The listing builds one solid part. Answer for the finished solid, in the listing's coordinates (mm). A direction names the side the tool comes from. Round coordinates to 2 decimals unless told otherwise and drop trailing zeros. Write each loop counter-clockwise with the first axis right and the second up, starting at its lowest first coordinate (ties: lowest second). Pieces come first, ordered by that corner, then holes. Notation, with made-up numbers: (-29.75, 32.25) - (24.25, 32.25) arc R16 ccw to (24.25, 54.25) - close; hole circle Ø6 at (-34.5, 40.25). An arc over 180 degrees is marked (long way). Answer as CSV lines item,"result". Start each with the question number.
Item 1: Which of the six approach directions +Z, -Z, +X, -X, +Y, -Y give full straight-line access (tool end or side, diameter ignored) to faces 1 (the flat face through (69.167, -0.231, 39.005)), 2 (the flat face through (8, 19.05, 28)), 3 (the flat face through (-51.3, -0.23, 20.22))?
Item 2: A cutting plane is placed at C-C on z = 50.5. Determine the outline of the cut face in (x, y), and give its area (3 significant figures).
Item 3: For a pull along Y with two mould halves and no side action, classify faces 4 (the flat face through (8, -19.05, 29)), 5 (the flat face through (11.1, -0.27, 9.39)), 6 (the flat face through (8, 16.51, 29)), 7 (the flat face through (8, -16.51, 29)) as pulls with the +Y half, pulls with the -Y half, needs draft (parallel to the pull), parting line crosses it, or undercut.
Item 4: A cutting plane is placed at A-A on z = 17. Determine the outline of the cut face in (x, y).
Item 5: Straight lines are drawn through the part: line 1 along Y through (x, z) = (-25, 39); line 2 along X through (y, z) = (9.5, 35); line 3 along X through (y, z) = (-4.5, 33). For each, find the intervals that lie inside material, in ascending order. Write a range as [from, to].
Item 6: A cutting plane is placed at B-B on y = 2. Determine the outline of the cut face in (x, z) (3 decimals), and give its area (3 significant figures).
Item 7: A cutting plane is placed at D-D on z = 31. Determine the outline of the cut face in (x, y).
Item 8: Flat-ended cylindrical pins translate along their axes: pin 1 (1.5 mm diameter, centred on x = 32, y = -13, fed in from -Z); pin 2 (3 mm diameter, centred on x = -29.5, y = -0.5, fed in from -Z); pin 3 (6 mm diameter, centred on x = -29, y = 5, fed in from -Z). Find the tip coordinate at first contact, or state that the pin passes through.
```python
from build123d import *

# Parameters (mm, degrees)
F1_DEPTH = 19.05
F2_W     = 121.92
F2_H     = 2.54
F3_DEPTH = 35.56


with BuildPart() as f1:
    # F0 (on Front) → F1 (new body, symmetric)
    with BuildSketch(Plane.XZ):
        Polygon((-56.515, 37.6689364729), (-50.8, 0), (74.7631215764, 19.05), (69.0481215764, 56.7189364729), (66.5368591448, 56.3379364729), (71.8708591448, 21.1802624315), (-48.6697375685, 2.8922624315), (-54.0037375685, 38.0499364729), align=None)
    extrude(amount=F1_DEPTH, both=True)

    # F2 (on face) → F3 (join)
    with BuildSketch(Plane(origin=(-1.524, 0, 10.0450497261), x_dir=(0.9886859967, 0, 0.15), z_dir=(-0.15, 0, 0.9886859967))):
        with Locations((13.2747513695, 17.78)):
            Rectangle(F2_W, F2_H)
        with Locations((13.2747513695, -17.78)):
            Rectangle(F2_W, F2_H)
    extrude(amount=F3_DEPTH)


solid = f1.part
```
Geometry says:
1,face 1,"none"
1,face 2,"+Z, -Z, +X, -X, +Y"
1,face 3,"+Z"
2,outline,"(28.06, -19.05) - (69.99, -19.05) - (69.99, 19.05) - (28.06, 19.05) - (28.06, 16.51) - (67.42, 16.51) - (67.42, -16.51) - (28.06, -16.51) - close"
2,area,"298 mm^2"
3,face 4,"pulls with the -Y half"
3,face 5,"needs draft"
3,face 6,"undercut"
3,face 7,"undercut"
4,outline,"(-53.38, -19.05) - (61.25, -19.05) - (61.25, 19.05) - (-53.38, 19.05) - close; hole (-50.81, -16.51) - (44.32, -16.51) - (44.32, 16.51) - (-50.81, 16.51) - close"
5,line 1,"y = [-19.05, -16.51], [16.51, 19.05]"
5,line 2,"x = [-56.11, -53.54], [69.77, 72.34]"
5,line 3,"x = [-55.81, -53.24], [70.08, 72.65]"
6,outline,"(-56.515, 37.669) - (-50.8, 0) - (74.763, 19.05) - (69.048, 56.719) - (66.537, 56.338) - (71.871, 21.18) - (-48.67, 2.892) - (-54.004, 38.05) - close"
6,area,"503 mm^2"
7,outline,"(-55.5, -19.05) - (72.95, -19.05) - (72.95, 19.05) - (-55.5, 19.05) - close; hole (-52.93, -16.51) - (70.38, -16.51) - (70.38, 16.51) - (-52.93, 16.51) - close"
8,pin 1,"stops at z = 12.45"
8,pin 2,"stops at z = 3"
8,pin 3,"stops at z = 2.85"
